For this review, take the finished solid that the model builds, in its own axes (mm). A direction names the side the tool comes from. Round coordinates to 2 decimals unless told otherwise and drop trailing zeros. Loops run counter-clockwise (first coordinate to the right, second up) from the corner with the lowest first, then second, coordinate; pieces in that order, holes last. Notation, with made-up numbers: (-12.75, 57) -> (-6.75, 57) arc R24 ccw to (-6.75, 91) -> close; hole circle Ø9 at (52.25, 79). An arc over 180 degrees is marked (long way). Write each question's results on one line, items separated by ' | '.
```python
from build123d import *

# Parameters (mm, degrees)
F0_W     = 78
F0_H     = 17.5
F1_DEPTH = 2
F2_W     = 36
F2_H     = 2.7
F2_W_2   = 2
F2_H_2   = 2.1
F3_DEPTH = 5
F4_W     = 2
F4_H     = 2.1
F5_DEPTH = 1
F6_SIZE  = 0.99999


# Not quite as in the source:
# - a fillet or chamfer is up to 0.001 mm smaller than in the source, because OpenCascade refuses the exact size


with BuildPart() as f1:
    # F0 (on Top) → F1 (new body)
    with BuildSketch(Plane.XY):
        Rectangle(F0_W, F0_H)
    extrude(amount=F1_DEPTH)

    # F2 (on face) → F3 (join)
    with BuildSketch(Plane.XY.offset(2)):
        Polygon((-13.5, -3.95), (-13.5, -4.75), (23.5, -4.75), (23.5, -3.95), (23.5, -1.85), (23.5, -1.05), (-13.5, -1.05), (-13.5, -1.85), align=None)
        with Locations((5, -2.9)):
            Rectangle(F2_W, F2_H, mode=Mode.SUBTRACT)
        with Locations((-14.5, -2.9)):
            Rectangle(F2_W_2, F2_H_2)
        with Locations((24.5, -2.9)):
            Rectangle(F2_W_2, F2_H_2)
    extrude(amount=F3_DEPTH)

    # F4 (on face) → F5 (join)
    with BuildSketch(Plane.XY.offset(7)):
        with Locations((-14.5, -2.9)):
            Rectangle(F4_W, F4_H)
        with Locations((24.5, -2.9)):
            Rectangle(F4_W, F4_H)
    extrude(amount=F5_DEPTH)

    # F6 (size 1 in the source; OpenCascade refuses exactly that, so slightly less here)
    f6_edges = [f1.edges().sort_by_distance(p)[0] for p in [
        (-15.5, -2.9, 8),
        (-14.5, -1.85, 8),
        (-13.5, -2.9, 8),
        (-14.5, -3.95, 8),
        (24.5, -1.85, 8),
        (23.5, -2.9, 8),
        (25.5, -2.9, 8),
        (24.5, -3.95, 8),
    ]]
    chamfer(f6_edges, length=F6_SIZE)


solid = f1.part
```
1. Consider section C-C (y = -5.75). State the section outline as (x, z) points, plus the area to 3 significant figures.
Values found:
outline: (-39, 0) -> (39, 0) -> (39, 2) -> (-39, 2) -> close | area: 156 mm2
2. To check wall thickness, follow probe 1 along Y at (x, z) = (-5.5, 3.25); probe 2 along Z at (x, y) = (23, 4); probe 3 along X at (y, z) = (-3.25, 7.5). State the ranges of each line that lie inside material, in increasing order.
Values found:
probe 1: y = -4.75 to -4.25, -1.55 to -1.05 | probe 2: z = 0 to 2 | probe 3: x = -15 to -14, 24 to 25
3. Consider section B-B (x = 6). State the section outline as (y, z) points, plus the area to 3 significant figures.
Values found:
outline: (-8.75, 0) -> (8.75, 0) -> (8.75, 2) -> (-1.05, 2) -> (-1.05, 7) -> (-1.55, 7) -> (-1.55, 2) -> (-4.25, 2) -> (-4.25, 7) -> (-4.75, 7) -> (-4.75, 2) -> (-8.75, 2) -> close | area: 40.0 mm2
4. Consider section D-D (x = -26.5). State the section outline as (y, z) points, plus the area to 3 significant figures.
Values found:
outline: (-8.75, 0) -> (8.75, 0) -> (8.75, 2) -> (-8.75, 2) -> close | area: 35.0 mm2
5. For pin 1 (1.6 mm diameter, centred on x = 24.5, z = 4, fed in from -Y); pin 2 (8 mm diameter, centred on x = 14, y = -3, fed in from +Z); pin 3 (0.6 mm diameter, centred on y = -4.5, z = 4, fed in from -X), all flat-tipped, find the tip position at first contact; note any pin that passes through.
Values found:
pin 1: stops at y = -3.95 | pin 2: stops at z = 7 | pin 3: stops at x = -13.5
6. Consider section A-A (z = 4). State the section outline as (x, y) points, plus the area to 3 significant figures.
Values found:
outline: (-15.5, -3.95) -> (-13.5, -3.95) -> (-13.5, -4.75) -> (23.5, -4.75) -> (23.5, -3.95) -> (25.5, -3.95) -> (25.5, -1.85) -> (23.5, -1.85) -> (23.5, -1.05) -> (-13.5, -1.05) -> (-13.5, -1.85) -> (-15.5, -1.85) -> close; hole (-13, -4.25) -> (23, -4.25) -> (23, -1.55) -> (-13, -1.55) -> close | area: 48.1 mm2
7. Tool access review of faces 1 (the face through (-15.5, -3, 4)), 2 (the face through (5, -1.55, 4)), 3 (the face through (24, -1.85, 4)), 4 (the face through (5, -4.75, 4)): name each direction out of +Z, -Z, +X, -X, +Y, -Y from which nothing blocks a thin tool from reaching the whole face with its end or side.
Values found:
face 1: +Z, -X, +Y, -Y | face 2: +Z | face 3: +Z, +X, +Y | face 4: +Z, +X, -X, -Y
8. Draft analysis for pull direction X (two halves, no side actions). For faces 5 (the face through (25.5, -3, 4)), 6 (the face through (5, -3, 2)), 7 (the face through (5, -1.05, 4)), state which applies: released by +X, released by -X, zero draft, split by the parting line, or undercut.
Values found:
face 5: released by +X | face 6: undercut | face 7: zero draft
